Model file for the job. Use its own axes, mm. A direction names the side the tool comes from. Give positions to 0.01 mm unless a question says otherwise; leave off trailing zeros. Order: outer loops, then holes, each group sorted by start corner. A loop starts at its lowest first (then second) coordinate and runs counter-clockwise, first axis right, second up. Notation, with made-up numbers: M 8,-32 L 25,-32 A6 ccw 25,-21 Z; hole C 37,-20.75 d11. An arc over 180 degrees is marked long. Return JSON: item names as keys, results as strings. Group by question number.
1. Slice it at C-C on z = 4. List the corners of the cut face in (x, y), then the cut area to 3 significant figures.
2. Slice it at D-D on z = 1.5. List the corners of the cut face in (x, y).
3. Pin check, flat tips, straight feed: pin 1 (1.5 mm diameter, centred on y = -1, z = 3, fed in from -X); pin 2 (1.8 mm diameter, centred on x = 0, y = 0, fed in from -Z); pin 3 (1.5 mm diameter, centred on y = -2, z = -1, fed in from -X); pin 4 (3 mm diameter, centred on x = 0, y = 1, fed in from +Z). Stop position of each tip, or through.
4. 3-axis set-ups, long thin cutter, end or side, ignore diameter. For faces 1 (the face through (0, 0, -1)), 2 (the face through (2, 1, -5)): which of +Z, -Z, +X, -X, +Y, -Y reach the whole face in a straight line?
5. Two-plate mould, pull along X, no slides. Class faces 3 (the face through (1.624, 0.511, 3.028)), 4 (the face through (0, 0, 1)), 5 (the face through (-0.54, -2.44, 0.07)), 6 (the face through (2, 1, 5)): released by +X, released by -X, zero draft, split by the parting line, or undercut.
6. Wall check: probe 1 along Y at (x, z) = (0, 1.05) (3 decimals); probe 2 along Z at (x, y) = (-0.3, -0.5); probe 3 along X at (y, z) = (-2, 0). Give the ranges that are in metal, low to high. Write a range as [from, to].
from build123d import *

# Parameters (mm, degrees)
F0_R     = 1.5
F1_DEPTH = 1
F0_R_2   = 2.5
F2_DEPTH = 5
F3_SIZE2 = 0.39999
F3_SIZE  = 3.99999
F4_SIZE2 = 3.99999
F4_SIZE  = 0.39999


# Not quite as in the source:
# - a fillet or chamfer is up to 0.001 mm smaller than in the source, because OpenCascade refuses the exact size


with BuildPart() as f1:
    # F0 (on Top) → F1 (new body, symmetric)
    with BuildSketch(Plane.XY):
        Circle(F0_R)
    extrude(amount=F1_DEPTH, both=True)

    # F0 (on Top) → F2 (join, symmetric)
    with BuildSketch(Plane.XY):
        Circle(F0_R_2)
        Circle(F0_R, mode=Mode.SUBTRACT)
    extrude(amount=F2_DEPTH, both=True)

    # F3 (size 4 and 0.4 in the source; OpenCascade refuses exactly that, so slightly less here)
    f3_edges = [f1.edges().sort_by_distance(p)[0] for p in [
        (-1.5, 0, 5),
    ]]
    f3_side = f1.faces().sort_by_distance((-1.5, 0, 3))[0]
    chamfer(f3_edges, length=F3_SIZE, length2=F3_SIZE2, reference=f3_side)

    # F4 (size 0.4 and 4 in the source; OpenCascade refuses exactly that, so slightly less here)
    f4_edges = [f1.edges().sort_by_distance(p)[0] for p in [
        (-1.5, 0, -5),
    ]]
    f4_side = f1.faces().sort_by_distance((-2.429289, 0, -5))[0]
    chamfer(f4_edges, length=F4_SIZE, length2=F4_SIZE2, reference=f4_side)


solid = f1.part
Result:
{
 "1": {"outline": "C 0,0 d5; hole C 0,0 d3.6", "area": "9.46 mm2"},
 "2": {"outline": "C 0,0 d5; hole C 0,0 d3.1"},
 "3": {"pin 1": "stops at x = -2.49", "pin 2": "stops at z = -1", "pin 3": "stops at x = -2.17", "pin 4": "stops at z = 5"},
 "4": {"face 1": "-Z", "face 2": "-Z, +X, -X, +Y, -Y"},
 "5": {"face 3": "undercut", "face 4": "undercut", "face 5": "split by the parting line", "face 6": "zero draft"},
 "6": {"probe 1": "y = [-2.5, -1.505], [1.505, 2.5]", "probe 2": "z = [-1, 1]", "probe 3": "x = [-1.5, 1.5]"}
}
